```python
from build123d import *

# Parameters (mm, degrees)
SKETCH3_R      = 12.5
EXTRUDE1_DEPTH = 0.5


with BuildPart() as part:
    # Sketch3 → Extrude1 (new, symmetric)
    with BuildSketch(Plane(origin=(0, 0, 0), x_dir=(0, 0, -1), z_dir=(1, 0, 0))):
        with BuildLine():
            ThreePointArc((-36.207031651, 9.762215886), (-4.923734004, -37.175352634), (37.5, 0))
            add(Edge.make_bspline(
                [(54.652290082, 423.825278241), (52.509509177, 404.859584217), (61.688430189, 350.928455024), (93.740739008, 248.146468923), (40.812256209, 127.830390939), (37.5, 38.493002207), (37.5, 0)],
                knots=[0, 0, 0, 0, 0.133447201, 0.376558764, 0.731484898, 1, 1, 1, 1], degree=3))
            ThreePointArc((54.652290082, 423.825278241), (-10.84310867, 483.920561889), (-48.017058979, 403.179074456))
            add(Edge.make_bspline(
                [(-48.017058979, 403.179074456), (-41.112444302, 390.817857106), (-27.905320028, 336.914546659), (-50.20843212, 219.173527848), (-32.204632677, 102.502128563), (-32.423669788, 23.794306992), (-36.207031651, 9.762215886)],
                knots=[0, 0, 0, 0, 0.106358982, 0.411206468, 0.890017974, 1, 1, 1, 1], degree=3))
        make_face()
        with Locations((0, 430)):
            Circle(SKETCH3_R, mode=Mode.SUBTRACT)
        Circle(SKETCH3_R, mode=Mode.SUBTRACT)
    extrude(amount=EXTRUDE1_DEPTH, both=True)


solid = part.part
```
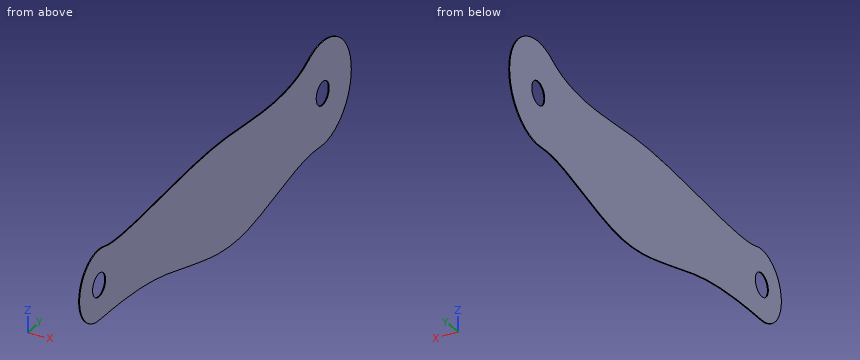
Input: part model. Units: mm. Frame: model coordinates. Coordinates: 2 decimals unless noted, no trailing zeros. Write each loop counter-clockwise with the first axis right and the second up, starting at its lowest first coordinate (ties: lowest second). Pieces come first, ordered by that corner, then holes. Notation, with made-up numbers: M 59,14 L 115,14 A20 cw 115,43 Z; hole C 34,35 d7. An arc over 180 degrees is marked long. Use one line per item in the form item = value.
Q1. Material intervals for probe 1 along Y at (x, z) = (-0.4, -9); probe 2 along Y at (x, z) = (0.3, 0); probe 3 along Z at (x, y) = (-0.15, 438), sorted ascending. Write a range as from..to.
Answer below:
probe_1 = -36.4..-8.67, 8.67..421.33, 438.67..484.26
probe_2 = -37.5..-12.5, 12.5..417.5, 442.5..485
probe_3 = -54.42..-9.6, 9.6..54.42
Q2. Section D-D (z = 19). Return loops of the section in (x, y), plus the area to 3 significant figures.
Answer below:
outline = M -0.5,-32.33 L 0.5,-32.33 L 0.5,481.61 L -0.5,481.61 Z
area = 514 mm²
Q3. Section B-B (y = 430). Return loops of the section in (x, z).
Answer below:
outline = M -0.5,-55 L 0.5,-55 L 0.5,-12.5 L -0.5,-12.5 Z; M -0.5,12.5 L 0.5,12.5 L 0.5,55 L -0.5,55 Z
Q4. Section A-A (z = 0). Return loops of the section in (x, y).
Answer below:
outline = M -0.5,-37.5 L 0.5,-37.5 L 0.5,-12.5 L -0.5,-12.5 Z; M -0.5,12.5 L 0.5,12.5 L 0.5,417.5 L -0.5,417.5 Z; M -0.5,442.5 L 0.5,442.5 L 0.5,485 L -0.5,485 Z
Q5. Section C-C (x = -0.25). Count the separate pieces of the cut face and the enclosed holes in it, plus the area to 3 significant figures.
Answer below:
separate_pieces = 1
enclosed_holes = 2
area = 47,600 mm²
